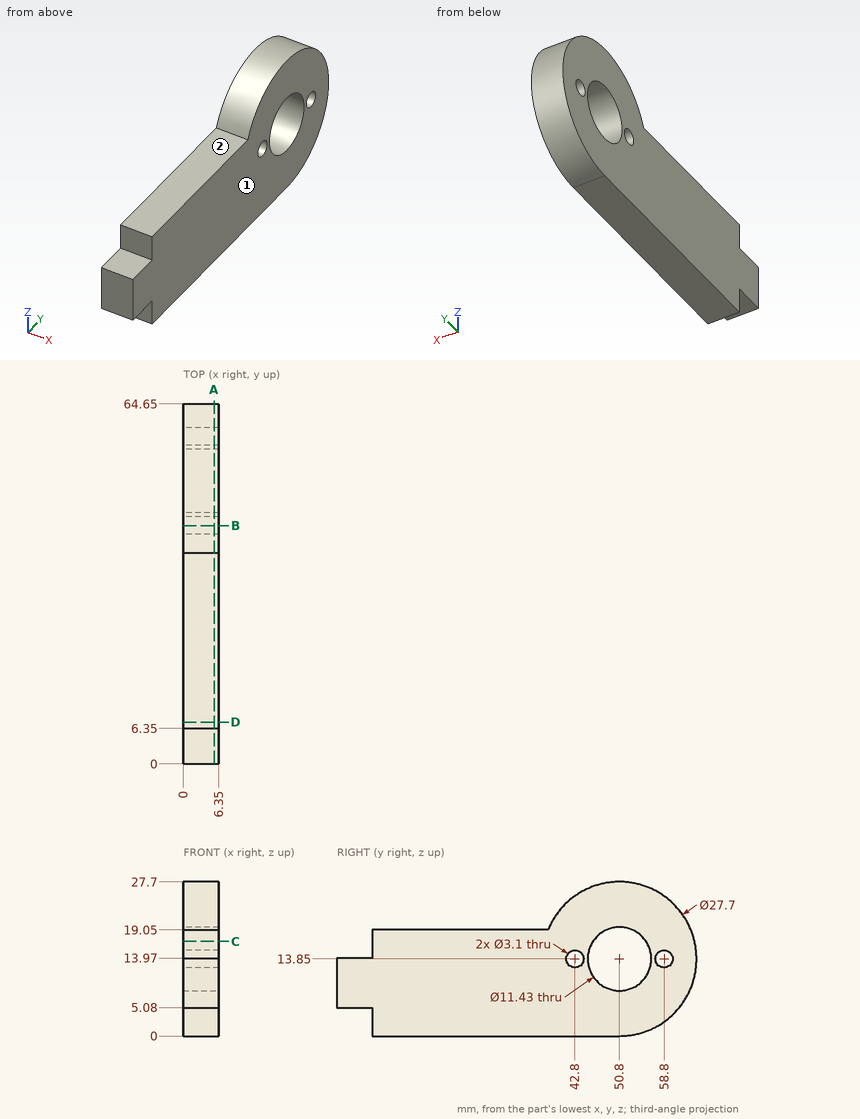
Could you check a few things on this drawing? It's one solid part, dimensions in mm from its lowest x, y, z. A direction names the side the tool comes from. Give positions to 0.01 mm unless a question says otherwise; leave off trailing zeros. Order: outer loops, then holes, each group sorted by start corner. A loop starts at its lowest first (then second) coordinate and runs counter-clockwise, first axis right, second up. Notation, with made-up numbers: (32, 47.5) - (55, 47.5) arc R32 ccw to (55, 86.5) - close; hole circle Ø3 at (30, 50). An arc over 180 degrees is marked (long way). Return JSON: item names as keys, results as strings. Group by question number.
Q1. Suppose I cut it at D-D, the plane y = 7.5. Please give me the cut outline in (x, z), and give its area (3 significant figures).
Q2. Please list where these lines run through material, in increasing order: line 1 along Y through (x, z) = (3, 13.85) (3 decimals); line 2 along Y through (x, z) = (5, 15); line 3 along Y through (x, z) = (1.75, 15.5). Write a range as [from, to].
Q3. Suppose I cut it at B-B, the plane y = 42.8. Please give me the cut outline in (x, z).
Q4. Will these pins go through, and if not, where does the flat tip stop? pin 1 Ø1.9 at (x, y) = (3, 21) entering from +Z; pin 2 Ø1.5 at (x, y) = (4.5, 57.5) entering from +Z; pin 3 Ø2.5 at (x, z) = (4.5, 3) entering from -Y.
Q5. Suppose I cut it at C-C, the plane z = 17. Please give me the cut outline in (x, y).
Q6. Suppose I cut it at A-A, the plane x = 5.5. Please give me the cut outline in (y, z) (3 decimals), and give its area (3 significant figures).
Q7. Which directions (+Z, -Z, +X, -X, +Y, -Y) give clear straight access to the entire face, cutting with the end or side of a thin tool? Please do the marked faces 1 and 2.
Resolved:
{
 "1": {"outline": "(0, 0) - (6.35, 0) - (6.35, 19.05) - (0, 19.05) - close", "area": "121 mm2"},
 "2": {"line 1": "y = [0, 41.25], [44.35, 45.085], [56.515, 57.25], [60.35, 64.65]", "line 2": "y = [6.35, 41.76], [43.84, 45.2], [56.4, 57.76], [59.84, 64.6]", "line 3": "y = [6.35, 45.33], [56.27, 64.55]"},
 "3": {"outline": "(0, 0) - (6.35, 0) - (6.35, 12.3) - (0, 12.3) - close; (0, 15.4) - (6.35, 15.4) - (6.35, 25.16) - (0, 25.16) - close"},
 "4": {"pin 1": "stops at z = 19.05", "pin 2": "stops at z = 26.36", "pin 3": "stops at y = 6.35"},
 "5": {"outline": "(0, 6.35) - (6.35, 6.35) - (6.35, 46.03) - (0, 46.03) - close; (0, 55.57) - (6.35, 55.57) - (6.35, 64.29) - (0, 64.29) - close"},
 "6": {"outline": "(0, 5.08) - (6.35, 5.08) - (6.35, 0) - (50.8, 0) arc R13.85 ccw (long way) to (37.963, 19.05) - (6.35, 19.05) - (6.35, 13.97) - (0, 13.97) - close; hole circle Ø3.1 at (42.8, 13.85); hole circle Ø11.43 at (50.8, 13.85); hole circle Ø3.1 at (58.8, 13.85)", "area": "1,170 mm2"},
 "7": {"face 1": "+Z, -Z, +X, +Y, -Y", "face 2": "+Z, +X, -X, -Y"}
}
